from build123d import *

# Parameters (mm, degrees)
SKETCH13_R              = 2.6
SKETCH13_R_2            = 3.55
BASE_FLANGE1_DEPTH      = 3.175
EDGE_FLANGE2_DEPTH      = 22.5
EDGE_FLANGE3_DEPTH      = 22.5
CUT_EXTRUDE3_DEPTH      = 944.619626468
CUT_EXTRUDE3_DEPTH_BACK = 944.619626468
EDGE_FLANGE4_DEPTH      = 147.523066449
CORNER_START            = 927.243279461
CORNER_RELIEF2_DEPTH    = 2.5875
CORNER_START_2          = 544.417983929
CORNER_RELIEF2_2_DEPTH  = 2.5875
CORNER_RELIEF3_DEPTH    = 2.5875
CORNER_START_3          = 689.353550378
CORNER_RELIEF3_2_DEPTH  = 2.5875


with BuildPart() as part:
    # Base-Flange1: sheet metal written as solids
    # Sketch13 → Base-Flange1 (new body)
    with BuildSketch(Plane(origin=(0, 0, 0), x_dir=(-1, 0, 0), z_dir=(0, 0, -1))):
        with BuildLine():
            Line((-547.592983929, 907.330779461), (-547.592983929, 814.180779461))
            ThreePointArc((-547.592983929, 814.180779461), (-553.450848305, 800.038643837), (-567.592983929, 794.180779461))
            Line((-567.592983929, 794.180779461), (-668.766050378, 794.180779461))
            ThreePointArc((-668.766050378, 794.180779461), (-682.908186002, 800.038643837), (-688.766050378, 814.180779461))
            Line((-688.766050378, 814.180779461), (-688.766050378, 907.330779461))
            Line((-688.766050378, 907.330779461), (-691.941050378, 907.330779461))
            Line((-691.941050378, 907.330779461), (-691.941050378, 929.830779461))
            Line((-691.941050378, 929.830779461), (-544.417983929, 929.830779461))
            Line((-544.417983929, 929.830779461), (-544.417983929, 907.330779461))
            Line((-544.417983929, 907.330779461), (-547.592983929, 907.330779461))
        make_face()
        with Locations((-681.766050378, 917.330779461)):
            Circle(SKETCH13_R, mode=Mode.SUBTRACT)
        with Locations((-618.179517153, 836.030779461)):
            Circle(SKETCH13_R_2, mode=Mode.SUBTRACT)
        with Locations((-554.592983929, 917.330779461)):
            Circle(SKETCH13_R, mode=Mode.SUBTRACT)
    extrude(amount=-BASE_FLANGE1_DEPTH)

    # Edge-Flange2: sheet metal written as solids
    # Edge-Flange2 section (on a plane across the edge) → Edge-Flange2 (add)
    with BuildSketch(Plane(origin=(695.116050378, 907.330779461, 3.175), x_dir=(-1, 0, 0), z_dir=(0, 1, 0))):
        with BuildLine():
            Line((-3.175, 3.175), (-3.175, 9.525))
            Line((-3.175, 9.525), (0, 9.525))
            Line((0, 9.525), (0, 3.175))
            ThreePointArc((0, 3.175), (0.92993597, 0.92993597), (3.175, 0))
            Line((3.175, 0), (3.175, -3.175))
            ThreePointArc((3.175, -3.175), (-1.315128061, -1.315128061), (-3.175, 3.175))
        make_face()
    extrude(amount=EDGE_FLANGE2_DEPTH)

    # Edge-Flange3: sheet metal written as solids
    # Edge-Flange3 section (on a plane across the edge) → Edge-Flange3 (add)
    with BuildSketch(Plane(origin=(541.242983929, 929.830779461, 3.175), x_dir=(1, 0, 0), z_dir=(0, -1, 0))):
        with BuildLine():
            Line((-3.175, 3.175), (-3.175, 9.525))
            Line((-3.175, 9.525), (0, 9.525))
            Line((0, 9.525), (0, 3.175))
            ThreePointArc((0, 3.175), (0.92993597, 0.92993597), (3.175, 0))
            Line((3.175, 0), (3.175, -3.175))
            ThreePointArc((3.175, -3.175), (-1.315128061, -1.315128061), (-3.175, 3.175))
        make_face()
    extrude(amount=EDGE_FLANGE3_DEPTH)

    # Sketch27 → Cut-Extrude3 (cut, two sides: drawn at the far end of the back side and taken through both)
    with BuildSketch(Plane(origin=(698.291050378, 0, 0), x_dir=(0, 0, -1), z_dir=(1, 0, 0)).offset(-CUT_EXTRUDE3_DEPTH_BACK)):
        with BuildLine():
            Line((-9.525, 911.558356296), (-9.525, 925.603202625))
            ThreePointArc((-9.525, 925.603202625), (-7.9375, 927.190702625), (-6.35, 925.603202625))
            Line((-6.35, 925.603202625), (-6.35, 911.558356296))
            ThreePointArc((-6.35, 911.558356296), (-7.9375, 909.970856296), (-9.525, 911.558356296))
        make_face()
    extrude(amount=CUT_EXTRUDE3_DEPTH + CUT_EXTRUDE3_DEPTH_BACK, mode=Mode.SUBTRACT)

    # Edge-Flange4: sheet metal written as solids
    # Edge-Flange4 section (on a plane across the edge) → Edge-Flange4 (add)
    with BuildSketch(Plane(origin=(544.417983929, 934.005779461, 0), x_dir=(0, -1, 0), z_dir=(1, 0, 0))):
        with BuildLine():
            Line((-3.175, 3.175), (-3.175, 45))
            Line((-3.175, 45), (0, 45))
            Line((0, 45), (0, 3.175))
            ThreePointArc((0, 3.175), (0.92993597, 0.92993597), (3.175, 0))
            Line((3.175, 0), (4.175, 0))
            Line((4.175, 0), (4.175, -3.175))
            Line((4.175, -3.175), (3.175, -3.175))
            ThreePointArc((3.175, -3.175), (-1.315128061, -1.315128061), (-3.175, 3.175))
        make_face()
    extrude(amount=EDGE_FLANGE4_DEPTH)

    # Corner Relief2: read off the stored shape, not the designer's step
    # Corner Relief2 outline → Corner Relief2 (cut)
    with BuildSketch(Plane(origin=(0, 0, 0), x_dir=(1, 0, 0), z_dir=(0, 1, 0)).offset(CORNER_START)):
        with BuildLine():
            Line((541.013027484, -0.990077276), (542.715505707, -3.670038638))
            ThreePointArc((542.715505707, -3.670038638), (543.531488674, -3.301270566), (544.417983929, -3.175))
            Line((544.417983929, -3.175), (544.417983929, 0))
            ThreePointArc((544.417983929, 0), (542.644993418, -0.252541132), (541.013027484, -0.990077276))
        make_face()
    extrude(amount=CORNER_RELIEF2_DEPTH, mode=Mode.SUBTRACT)

    # Corner Relief2 2 outline → Corner Relief2 2 (cut)
    with BuildSketch(Plane.YZ.offset(CORNER_START_2)):
        with BuildLine():
            Line((930.830779461, 3.175), (927.243279461, 3.175))
            Line((927.243279461, 3.175), (927.243279461, 0))
            Line((927.243279461, 0), (930.830779461, 0))
            ThreePointArc((930.830779461, 0), (931.379229895, -0.047728486), (931.911191064, -0.189478979))
            Line((931.911191064, -0.189478979), (932.991602668, 2.796042042))
            ThreePointArc((932.991602668, 2.796042042), (931.92768033, 3.079543028), (930.830779461, 3.175))
        make_face()
    extrude(amount=CORNER_RELIEF2_2_DEPTH, mode=Mode.SUBTRACT)

    # Corner Relief3: read off the stored shape, not the designer's step
    # Corner Relief3 outline → Corner Relief3 (cut)
    with BuildSketch(Plane(origin=(0, 0, 0), x_dir=(1, 0, 0), z_dir=(0, 1, 0)).offset(CORNER_START)):
        with BuildLine():
            ThreePointArc((691.941050378, -3.175), (692.827545633, -3.301270566), (693.6435286, -3.670038638))
            Line((693.6435286, -3.670038638), (695.346006823, -0.990077276))
            ThreePointArc((695.346006823, -0.990077276), (693.714040889, -0.252541132), (691.941050378, 0))
            Line((691.941050378, 0), (691.941050378, -3.175))
        make_face()
    extrude(amount=CORNER_RELIEF3_DEPTH, mode=Mode.SUBTRACT)

    # Corner Relief3 2 outline → Corner Relief3 2 (cut)
    with BuildSketch(Plane.YZ.offset(CORNER_START_3)):
        with BuildLine():
            Line((930.830779461, 3.175), (927.243279461, 3.175))
            Line((927.243279461, 3.175), (927.243279461, 0))
            Line((927.243279461, 0), (930.830779461, 0))
            ThreePointArc((930.830779461, 0), (931.379229895, -0.047728486), (931.911191064, -0.189478979))
            Line((931.911191064, -0.189478979), (932.991602668, 2.796042042))
            ThreePointArc((932.991602668, 2.796042042), (931.92768033, 3.079543028), (930.830779461, 3.175))
        make_face()
    extrude(amount=CORNER_RELIEF3_2_DEPTH, mode=Mode.SUBTRACT)


solid = part.part
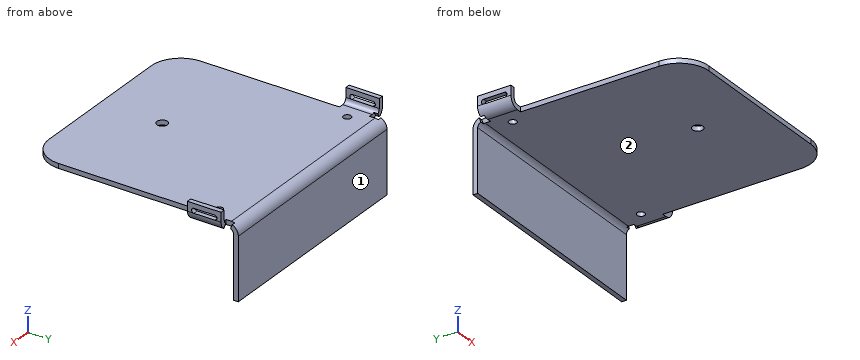
Part model, mm, in its own coordinate system. Face numbers are marked on the shaded views. A direction names the side the tool comes from. Give positions to 0.01 mm unless a question says otherwise; leave off trailing zeros. Write each loop counter-clockwise with the first axis right and the second up, starting at its lowest first coordinate (ties: lowest second). Pieces come first, ordered by that corner, then holes.
1) Pin check, flat tips, straight feed: pin 1 (12.5 mm diameter, centred on x = 615, z = -15.5, fed in from -Y); pin 2 (6 mm diameter, centred on y = 934.5, z = -29, fed in from -X); pin 3 (4 mm diameter, centred on x = 693, z = 2.5, fed in from +Y); pin 4 (4.5 mm diameter, centred on x = 554.59, y = 917.33, fed in from +Z). Stop position of each tip, or through.
Resolved:
pin 1: stops at y = 934.01
pin 2: stops at x = 544.42
pin 3: stops at y = 935.78
pin 4: passes through
2) Probe L1, parallel to Z at x = 600, y = 809 (3 decimals); L2, parallel to Y at x = 666, z = -6; L3, parallel to Y at x = 686.5, z = -2.5. List the from-to ranges inside material, lowest first.
Resolved:
L1: z = 0 to 3.175
L2: y = 934.01 to 937.18
L3: y = 933.93 to 937.14
3) Cut at C-C on z = -31.5. Write the cut outline in (x, y).
Resolved:
outline: (544.42, 934.01) - (691.94, 934.01) - (691.94, 937.18) - (544.42, 937.18) - close
4) Cut at B-B on x = 555. Write the cut outline in (y, z) (3 decimals).
Resolved:
outline: (798.643, 0) - (914.763, 0) - (914.763, 3.175) - (798.643, 3.175) - close; (919.899, 0) - (930.831, 0) arc R3.175 cw to (934.006, -3.175) - (934.006, -45) - (937.181, -45) - (937.181, -3.175) arc R6.35 ccw to (930.831, 3.175) - (919.899, 3.175) - close
5) Which spindle directions (+Z, -Z, +X, -X, +Y, -Y) get a long thin tool onto all of the face, cutting with end or side? Do the marked faces 1 and 2. Say none if no direction does.
Resolved:
face 1: +Z, -Z, +X, -X, +Y
face 2: -Z, +X, -X, -Y
6) Cut at A-A on x = 577. Write the cut outline in (y, z) (3 decimals), then the cut area to 3 significant figures.
Resolved:
outline: (794.181, 0) - (930.831, 0) arc R3.175 cw to (934.006, -3.175) - (934.006, -45) - (937.181, -45) - (937.181, -3.175) arc R6.35 ccw to (930.831, 3.175) - (794.181, 3.175) - close
area: 590 mm2
7) Cut at D-D on y = 899.5. Write the cut outline in (x, z) (3 decimals), then the cut area to 3 significant figures.
Resolved:
outline: (547.593, 0) - (688.766, 0) - (688.766, 3.175) - (547.593, 3.175) - close
area: 448 mm2
